The model under review builds one solid part; all positions refer to its coordinate system, in mm. A direction names the side the tool comes from. Round coordinates to 2 decimals unless told otherwise and drop trailing zeros. Order: outer loops, then holes, each group sorted by start corner. A loop starts at its lowest first (then second) coordinate and runs counter-clockwise, first axis right, second up.
1) Machinability: for faces 1 (the face through (1003, -1.524, -57)), 2 (the face through (538.497, -3.441, -15.497)), 3 (the face through (1003, 0, -57)), 4 (the face through (124.865, -0.751, -93.244)), 5 (the face through (0, 9, -98)), which of the approach directions +Z, -Z, +X, -X, +Y, -Y give a long, thin tool a straight path to every point of the face, cutting with its end or side? Answer none if there is none.
2) Consider section C-C (x = 781.5). Give the boundary of the cut face in (y, z) (3 decimals), then the cut area to 3 significant figures.
3) Mouldability with a two-part tool opening along Z and no side actions: class faces 6 (the face through (967.335, -0.751, -93.244)), 7 (the face through (1059, -0.8, -96.5)), 8 (the face through (1092.2, 9, -98)) as pulls with the +Z half, pulls with the -Z half, needs draft (parallel to the pull), parting line crosses it, or undercut.
4) Consider section A-A (z = 35.5). Give the boundary of the cut face in (x, y), then the cut area to 3 significant figures.
5) Clearance check with flat-ended pins moving along their axes: P1, Ø0.8, axis at x = 1078.5, y = -1, coming from the -Z side (3 decimals); P2, Ø6, axis at x = 218.5, y = 6.5, coming from the +Z side; P3, Ø1.5, axis at x = 182.5, z = -20.5, coming from the +Y side; P4, Ø12.5, axis at y = 0, z = 52.79, coming from the +X side. State where each tip first meets the part, or that it passes through.
6) Consider section B-B (z = -119.5). Give the boundary of the cut face in (x, y).
7) To check wall thickness, follow L1, parallel to X at y = -16.5, z = 53; L2, parallel to Z at x = 1.95, y = 0; L3, parallel to Z at x = 275, y = 0.5. State the ranges of each line that lie inside material, in increasing order.
from build123d import *

# Parameters (mm, degrees)
F0_R     = 15.875
F1_DEPTH = 1092.2
F0_W     = 76.2
F0_H     = 353.215248
F0_R_2   = 7.9375
F4_DEPTH = 3.048
F5_DEPTH = 1.524
F6_DEPTH = 1.524


with BuildPart() as f1:
    # F0 (on Right) → F1 (new body)
    with BuildSketch(Plane.YZ):
        Circle(F0_R)
    extrude(amount=F1_DEPTH)

    # F0 (on Right) → F4 (join)
    with BuildSketch(Plane.YZ):
        with Locations((0, -100.805804)):
            Rectangle(F0_W, F0_H)
        with Locations((0, -252.013428)):
            Circle(F0_R_2, mode=Mode.SUBTRACT)
        with Locations((0, -99.613428)):
            Circle(F0_R_2, mode=Mode.SUBTRACT)
        Circle(F0_R, mode=Mode.SUBTRACT)
        with Locations((0, 52.786572)):
            Circle(F0_R_2, mode=Mode.SUBTRACT)
    extrude(amount=F4_DEPTH)

    # F2 (on Front) → F5 (join)
    with BuildSketch(Plane.XZ):
        with BuildLine():
            Line((228.6, 0), (0, 0))
            Line((0, 0), (0, -63.962556))
            ThreePointArc((0, -63.962556), (33.206645, -97.169202), (0, -130.375847))
            Line((0, -130.375847), (0, -168.275))
            Line((0, -168.275), (23.993986, -168.275))
            Line((23.993986, -168.275), (228.6, -16.082697))
            Line((228.6, -16.082697), (228.6, 0))
        make_face()
    extrude(amount=F5_DEPTH)

    # F2 (on Front) → F6 (join)
    with BuildSketch(Plane.XZ):
        with BuildLine():
            Line((228.6, 0), (0, 0))
            Line((0, 0), (0, -63.962556))
            ThreePointArc((0, -63.962556), (33.206645, -97.169202), (0, -130.375847))
            Line((0, -130.375847), (0, -168.275))
            Line((0, -168.275), (23.993986, -168.275))
            Line((23.993986, -168.275), (228.6, -16.082697))
            Line((228.6, -16.082697), (228.6, 0))
        make_face()
    extrude(amount=F6_DEPTH)

    # F7: F1 across plane


with BuildPart() as f1_1:
    add(f1.part)
    add(f1.part.mirror(Plane.YZ.offset(546.1)))


solid = f1_1.part
Answer below:
1. face 1: -Z, -Y
1. face 2: none
1. face 3: -Z, +Y
1. face 4: -Z, +Y, -Y
1. face 5: +Z, -Z, -X, +Y, -Y
2. outline: circle Ø31.75 at (0, 0)
2. area: 792 mm2
3. face 6: pulls with the -Z half
3. face 7: undercut
3. face 8: needs draft
4. outline: (0, -38.1) - (3.05, -38.1) - (3.05, 38.1) - (0, 38.1) - close; (1089.15, -38.1) - (1092.2, -38.1) - (1092.2, 38.1) - (1089.15, 38.1) - close
4. area: 465 mm2
5. P1: stops at z = -168.275
5. P2: stops at z = 15.48
5. P3: stops at y = 0
5. P4: passes through
6. outline: (0, -38.1) - (3.05, -38.1) - (3.05, 38.1) - (0, 38.1) - close; (24.58, -1.52) - (89.57, -1.52) - (89.57, 0) - (24.58, 0) - close; (1002.63, -1.52) - (1067.62, -1.52) - (1067.62, 0) - (1002.63, 0) - close; (1089.15, -38.1) - (1092.2, -38.1) - (1092.2, 38.1) - (1089.15, 38.1) - close
7. L1: x = 0 to 3.05, 1089.15 to 1092.2
7. L2: z = -277.41 to -259.95, -244.08 to -107.55, -91.68 to 44.85, 60.72 to 75.8
7. L3: z = -15.87 to 15.87
